Design review of the part built by this model. Coordinates are the model's own, in mm. A direction names the side the tool comes from. Coordinates: 2 decimals unless noted, no trailing zeros. Order: outer loops, then holes, each group sorted by start corner. A loop starts at its lowest first (then second) coordinate and runs counter-clockwise, first axis right, second up. Notation, with made-up numbers: M 19,55.25 L 76,55.25 A27 cw 76,84.25 Z; hole C 35,81.5 d8. An arc over 180 degrees is marked long. Answer as a JSON object with one key per item and string values.
from build123d import *

# Parameters (mm, degrees)
SKETCH_1_R               = 12
EXTRUDE_1_DEPTH          = 45
SKETCH_2_R               = 10
EXTRUDE_2_DEPTH          = 56
SKETCH_3_R               = 17.5
EXTRUDE_3_DEPTH          = 90
SKETCH_4_R               = 10
EXTRUDE_4_DEPTH          = 72
SKETCH_5_R               = 19.5
EXTRUDE_5_DEPTH          = 24
CUT_EXTRUDE_1_DEPTH      = 265.441865067
CUT_EXTRUDE_1_DEPTH_BACK = 2
SKETCH_6_OUTSIDE_W       = 94.744
SKETCH_6_OUTSIDE_H       = 94.744
SKETCH_6_OUTSIDE_R       = 18.5
SKETCH_7_R               = 22.5
EXTRUDE_6_DEPTH          = 6
SKETCH_8_R               = 13.5
EXTRUDE_7_DEPTH          = 147
SKETCH_10_OUTSIDE_W      = 129.982
SKETCH_10_OUTSIDE_H      = 129.982
SKETCH_10_OUTSIDE_R      = 9
CUT_EXTRUDE_2_DEPTH      = 27
SKETCH_11_OUTSIDE_W      = 129.982
SKETCH_11_OUTSIDE_H      = 129.982
SKETCH_11_OUTSIDE_R      = 8
CUT_EXTRUDE_3_DEPTH      = 2
CHAMFER_1_SIZE           = 1
CUT_EXTRUDE_4_DEPTH      = 412.23290238
CUT_EXTRUDE_4_DEPTH_BACK = 412.23290238
SKETCH_15_R              = 4


with BuildPart() as part:
    # 草图1 → 凸台-拉伸1 (new body)
    with BuildSketch(Plane.XY):
        with Locations(Location((0, 0, 0), (0, 0, 180))):
            Circle(SKETCH_1_R)
    extrude(amount=EXTRUDE_1_DEPTH)

    # 草图2 → 凸台-拉伸2 (add)
    with BuildSketch(Plane.XY.offset(45)):
        Circle(SKETCH_2_R)
    extrude(amount=EXTRUDE_2_DEPTH)

    # 草图3 → 凸台-拉伸3 (add)
    with BuildSketch(Plane.XY.offset(101)):
        with Locations(Location((0, 0, 0), (0, 0, 180))):
            Circle(SKETCH_3_R)
    extrude(amount=EXTRUDE_3_DEPTH)

    # 草图4 → 凸台-拉伸4 (add)
    with BuildSketch(Plane.XY.offset(191)):
        Circle(SKETCH_4_R)
    extrude(amount=EXTRUDE_4_DEPTH)

    # 草图5 → 凸台-拉伸5 (add)
    with BuildSketch(Plane.XY.offset(263)):
        Circle(SKETCH_5_R)
    extrude(amount=-EXTRUDE_5_DEPTH)

    # 草图6 outside → 切除-拉伸1 (cut, two sides: drawn at the far end of the back side and taken through both)
    with BuildSketch(Plane.XY.offset(263).offset(-CUT_EXTRUDE_1_DEPTH_BACK)):
        Rectangle(SKETCH_6_OUTSIDE_W, SKETCH_6_OUTSIDE_H)
        with Locations(Location((0, 0, 0), (0, 0, 180))):
            Circle(SKETCH_6_OUTSIDE_R, mode=Mode.SUBTRACT)
    extrude(amount=CUT_EXTRUDE_1_DEPTH + CUT_EXTRUDE_1_DEPTH_BACK, mode=Mode.SUBTRACT)

    # 草图7 → 凸台-拉伸6 (add)
    with BuildSketch(Plane.XY.offset(263)):
        Circle(SKETCH_7_R)
    extrude(amount=EXTRUDE_6_DEPTH)

    # 草图8 → 凸台-拉伸7 (add)
    with BuildSketch(Plane(origin=(0, 0, 263), x_dir=(-1, 0, 0), z_dir=(0, 0, -1))):
        Circle(SKETCH_8_R)
    extrude(amount=-EXTRUDE_7_DEPTH)

    # 草图10 outside → 切除-拉伸2 (cut)
    with BuildSketch(Plane.XY.offset(410)):
        Rectangle(SKETCH_10_OUTSIDE_W, SKETCH_10_OUTSIDE_H)
        Circle(SKETCH_10_OUTSIDE_R, mode=Mode.SUBTRACT)
    extrude(amount=-CUT_EXTRUDE_2_DEPTH, mode=Mode.SUBTRACT)

    # 草图11 outside → 切除-拉伸3 (cut)
    with BuildSketch(Plane.XY.offset(383)):
        Rectangle(SKETCH_11_OUTSIDE_W, SKETCH_11_OUTSIDE_H)
        Circle(SKETCH_11_OUTSIDE_R, mode=Mode.SUBTRACT)
    extrude(amount=CUT_EXTRUDE_3_DEPTH, mode=Mode.SUBTRACT)

    # 草图12 → 切除-旋转1 (revolve, cut)
    with BuildSketch(Plane(origin=(0, 0, 0), x_dir=(0, 0, -1), z_dir=(1, 0, 0)), mode=Mode.PRIVATE) as cut_revolve_1_sk:
        Polygon((-105.330127019, 17.5), (-101, 10), (-101, 17.5), align=None)
        Polygon((-191, 10), (-191, 17.5), (-186.669872981, 17.5), align=None)
    revolve(cut_revolve_1_sk.sketch.rotate(Axis((0, 0, 181.277430572), (0, 0, -1)), 90), axis=Axis((0, 0, 181.277430572), (0, 0, -1)), mode=Mode.SUBTRACT)

    # 倒角1
    chamfer_1_edges = [part.edges().sort_by_distance(p)[0] for p in [
        (12, 0, 0),
    ]]
    chamfer(chamfer_1_edges, length=CHAMFER_1_SIZE)

    # 草图14 → 切除-旋转2 (revolve, cut)
    with BuildSketch(Plane(origin=(0, 0, 0), x_dir=(0, 0, -1), z_dir=(1, 0, 0))):
        Polygon((-14, 8), (-23.293093205, 17.293093205), (-14, 17.293093205), align=None)
    revolve(axis=Axis((0, -18.394712119, 14), (0, 1, 0)), mode=Mode.SUBTRACT)

    # 草图15 → 切除-拉伸4 (cut, two sides: drawn at the far end of the back side and taken through both)
    with BuildSketch(Plane(origin=(0, 0, 0), x_dir=(1, 0, 0), z_dir=(0, 1, 0)).offset(-CUT_EXTRUDE_4_DEPTH_BACK)):
        with Locations(Location((0, -392, 0), (0, 0, 270))):
            Circle(SKETCH_15_R)
    extrude(amount=CUT_EXTRUDE_4_DEPTH + CUT_EXTRUDE_4_DEPTH_BACK, mode=Mode.SUBTRACT)


solid = part.part
1) Tool access review of faces 1 (the cylindrical face through (2.93, -13.18, 325.2)), 2 (the conical face through (-8.22, 6.31, 101.21)), 3 (the cylindrical face through (-2.539, 19.334, 250.154)): name each direction out of +Z, -Z, +X, -X, +Y, -Y from which nothing blocks a thin tool from reaching the whole face with its end or side.
Taken from the geometry:
{"face 1": "+Z", "face 2": "none", "face 3": "-Z"}
2) Insertion check: pin 1 Ø22.5 at (x, y) = (-9, -4) entering from +Z; pin 2 Ø8 at (y, z) = (1.5, 106.5) entering from +X; pin 3 Ø10 at (x, y) = (-12, -16.5) entering from +Z; pin 4 Ø8 at (x, z) = (-7, 170) entering from +Y. Each pin has a flat end and moves straight along its axis. Give the tip position at first contact, or say it passes through.
Taken from the geometry:
{"pin 1": "stops at z = 410", "pin 2": "stops at x = 17.5", "pin 3": "stops at z = 269", "pin 4": "stops at y = 17.24"}
3) Mouldability with a two-part tool opening along Z and no side actions: class faces 4 (the conical face through (-8.22, 6.31, 190.79)), 5 (the flat face through (10, -10, 269)), 6 (the flat face through (5, -9, 45)), 7 (the cylindrical face through (3.794, 17.084, 145.431)) as released by +Z, released by -Z, zero draft, split by the parting line, or undercut.
Taken from the geometry:
{"face 4": "undercut", "face 5": "released by +Z", "face 6": "undercut", "face 7": "zero draft"}
4) Add section B-B (z = 392). State the section outline as (x, y) points.
Taken from the geometry:
{"outline": "M -4,-8.06 L -4,8.06 A9 ccw Z; M 4,-8.06 A9 ccw 4,8.06 Z"}
5) To check wall thickness, follow L1, parallel to Z at x = 0, y = -5; L2, parallel to X at y = -1, z = 392; L3, parallel to Z at x = -10, y = -4.5. State the ranges of each line that lie inside material, in increasing order.
Taken from the geometry:
{"L1": "z = 0 to 388, 396 to 410", "L2": "x = -8.94 to -4, 4 to 8.94", "L3": "z = 0 to 45, 101.56 to 190.44, 239 to 383"}
6) Add section A-A (z = 162). State the section outline as (x, y) points, and give its area (3 significant figures).
Taken from the geometry:
{"outline": "C 0,0 d35", "area": "962 mm2"}
7) Add section C-C (z = 208.5). State the section outline as (x, y) points.
Taken from the geometry:
{"outline": "C 0,0 d20"}
